Could you check a few things on this drawing? It's one solid part, dimensions in mm from its lowest x, y, z. Coordinates: 2 decimals unless noted, no trailing zeros. Write each loop counter-clockwise with the first axis right and the second up, starting at its lowest first coordinate (ties: lowest second). Pieces come first, ordered by that corner, then holes. Notation, with made-up numbers: M 25.25,67 L 55.25,67 A21 ccw 55.25,77 Z; hole C 25,80.5 d2. An arc over 180 degrees is marked long. Use a Markdown table: item, result.
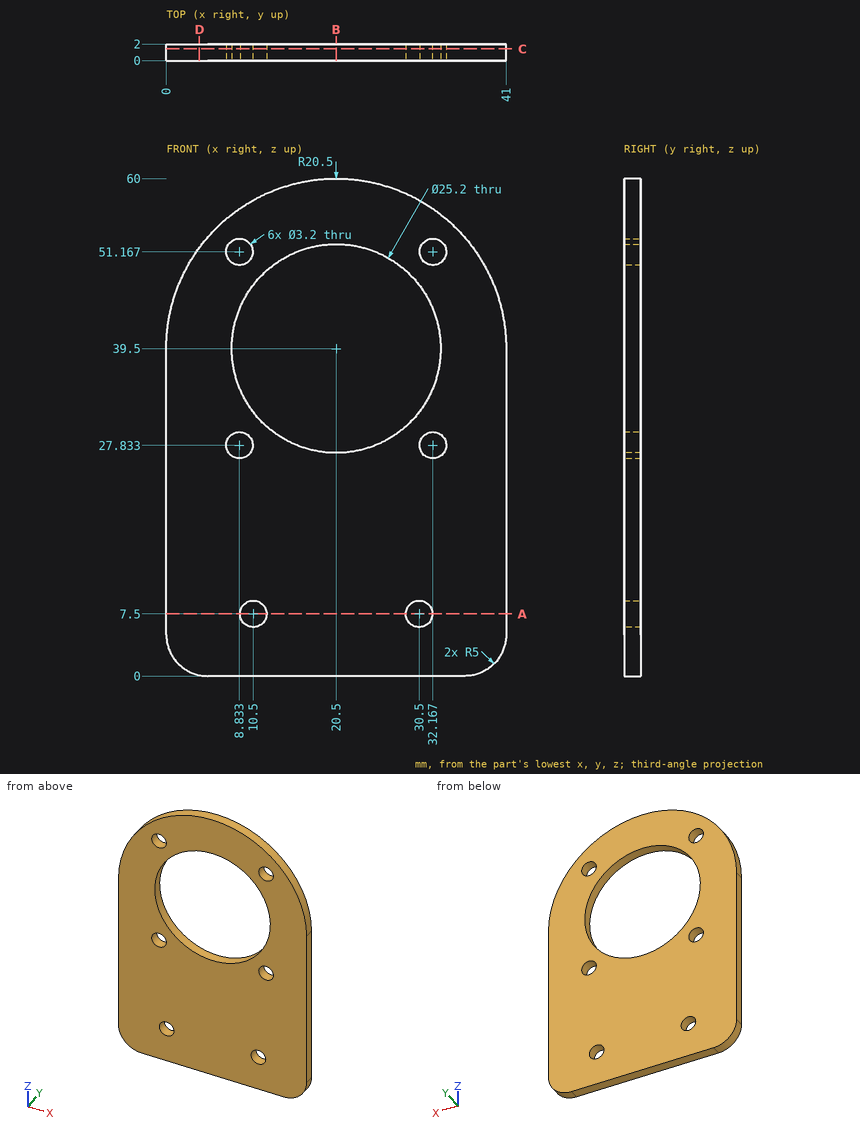
1. Suppose I cut it at D-D on x = 4. Write out the boundary of the cut face in (y, z) (1 decimal), and give its area (3 significant figures).
Answers follow:
| item | result |
|---|---|
| outline | M 0,0.1 L 2,0.1 L 2,51.7 L 0,51.7 Z |
| area | 103 mm2 |
2. Suppose I cut it at C-C on y = 1.4. Write out the boundary of the cut face in (x, z), and give its area (3 significant figures).
Answers follow:
| item | result |
|---|---|
| outline | M 0,5 A5 ccw 5,0 L 36,0 A5 ccw 41,5 L 41,39.5 A20.5 ccw 0,39.5 Z; hole C 8.83,27.83 d3.2; hole C 8.83,51.17 d3.2; hole C 20.5,39.5 d25.2; hole C 10.5,7.5 d3.2; hole C 30.5,7.5 d3.2; hole C 32.17,27.83 d3.2; hole C 32.17,51.17 d3.2 |
| area | 1,720 mm2 |
3. Suppose I cut it at A-A on z = 7.5. Write out the boundary of the cut face in (x, y).
Answers follow:
| item | result |
|---|---|
| outline | M 0,0 L 8.9,0 L 8.9,2 L 0,2 Z; M 12.1,0 L 28.9,0 L 28.9,2 L 12.1,2 Z; M 32.1,0 L 41,0 L 41,2 L 32.1,2 Z |
4. Suppose I cut it at B-B on x = 20.5. Write out the boundary of the cut face in (y, z).
Answers follow:
| item | result |
|---|---|
| outline | M 0,0 L 2,0 L 2,26.9 L 0,26.9 Z; M 0,52.1 L 2,52.1 L 2,60 L 0,60 Z |
5. Will these pins go through, and if not, where does the flat tip stop? pin 1 Ø3 at (x, z) = (8.83, 27.83) entering from -Y; pin 2 Ø1 at (y, z) = (1, 36.5) entering from -X.
Answers follow:
| item | result |
|---|---|
| pin 1 | passes through |
| pin 2 | stops at x = 0 |
6. I need wall thicknesses on probe 1 along X at (y, z) = (0.65, 7.5); probe 2 along X at (y, z) = (0.9, 39.5); probe 3 along Z at (x, y) = (7.5, 0.9). Which ranges of each line are inside material? Lowest first, please.
Answers follow:
| item | result |
|---|---|
| probe 1 | x = 0 to 8.9, 12.1 to 28.9, 32.1 to 41 |
| probe 2 | x = 0 to 7.9, 33.1 to 41 |
| probe 3 | z = 0 to 26.95, 28.72 to 50.28, 52.05 to 55.35 |
